Input: dimensioned drawing with shaded views. Units: mm. Origin: part minimum x, y, z. Coordinates: 2 decimals unless noted, no trailing zeros. Order: outer loops, then holes, each group sorted by start corner. A loop starts at its lowest first (then second) coordinate and runs counter-clockwise, first axis right, second up.
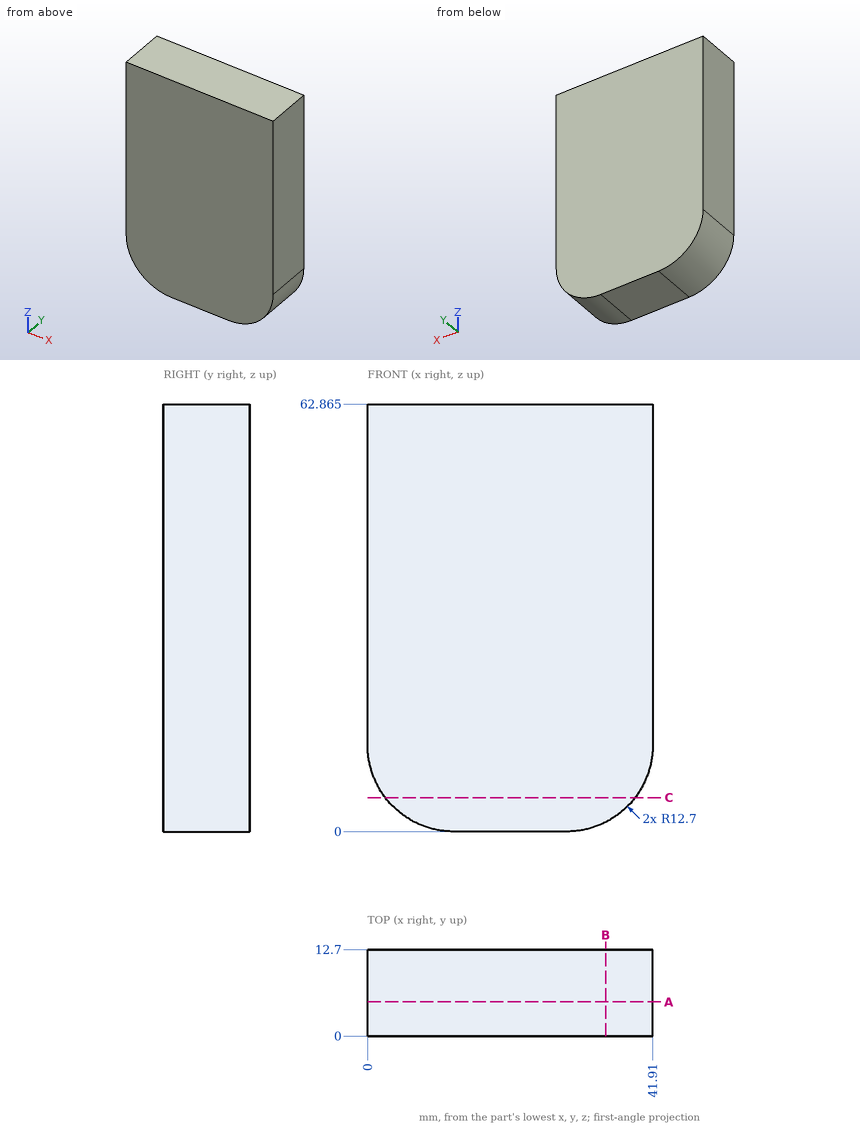
1. Section query C-C on z = 5. Return loops of the section in (x, y).
Findings:
outline: (2.6, 0) - (39.31, 0) - (39.31, 12.7) - (2.6, 12.7) - close
2. Section query A-A on y = 5. Return loops of the section in (x, z) (3 decimals).
Findings:
outline: (0, 12.7) arc R12.7 ccw to (12.7, 0) - (29.21, 0) arc R12.7 ccw to (41.91, 12.7) - (41.91, 62.865) - (0, 62.865) - close
3. Section query B-B on x = 35. Return loops of the section in (y, z) (3 decimals), plus the area to 3 significant figures.
Findings:
outline: (0, 1.397) - (12.7, 1.397) - (12.7, 62.865) - (0, 62.865) - close
area: 781 mm2
4. Ray query, line 1 (Z direction, x = 12.5, y = 2.25) (3 decimals); line 2 (Z direction, x = 33.5, y = 5.75) (3 decimals). Return the intervals inside material, ascending.
Findings:
line 1: z = 0.002 to 62.865
line 2: z = 0.747 to 62.865
5. Pin query (flat end, axial travel): P1, Ø3, axis at x = 16.5, y = 7, coming from the -Z side. Return the tip coordinate at first contact, or that it passes through.
Findings:
P1: stops at z = 0
